Source: three-view drawing plus pictorial views. Frame: mm from the lowest corner of the part. Give positions to 0.01 mm unless a question says otherwise; leave off trailing zeros. Order: outer loops, then holes, each group sorted by start corner. A loop starts at its lowest first (then second) coordinate and runs counter-clockwise, first axis right, second up. Notation, with made-up numbers: M 72.25,37.5 L 125.25,37.5 A12 ccw 125.25,49.5 Z; hole C -30,80.25 d8. An arc over 180 degrees is marked long. Use CSV: the item, a comma, the result in double quotes. Start each with the question number.
Item 1: First-contact query: pin 1 (1.5 mm diameter, centred on y = 3, z = 27, fed in from +X); pin 2 (2 mm diameter, centred on x = 109.5, z = 37.5, fed in from -Y). Flat tips, straight axial feed; report the tip coordinate or a pass-through.
Item 2: Ray query, probe 1 along Y at (x, z) = (116, 39.5); probe 2 along X at (y, z) = (4, 17); probe 3 along Y at (x, z) = (21, 33). Return the intervals inside material, ascending. Write a range as from..to.
Item 3: Pull-direction query (Y, two-part tool) for the marked faces 1, 2 and 3; classes: +Y half, -Y half, draft (parallel to the pull), parting line (faces both ways), or undercut.
Item 4: Section query D-D on x = 126. Return loops of the section in (y, z).
Item 5: Section query C-C on z = 38.5. Return loops of the section in (x, y).
Item 6: Section query B-B on z = 12.5. Return loops of the section in (x, y).
Item 7: Section query A-A on x = 87.5. Return loops of the section in (y, z), and give its area (3 significant figures).
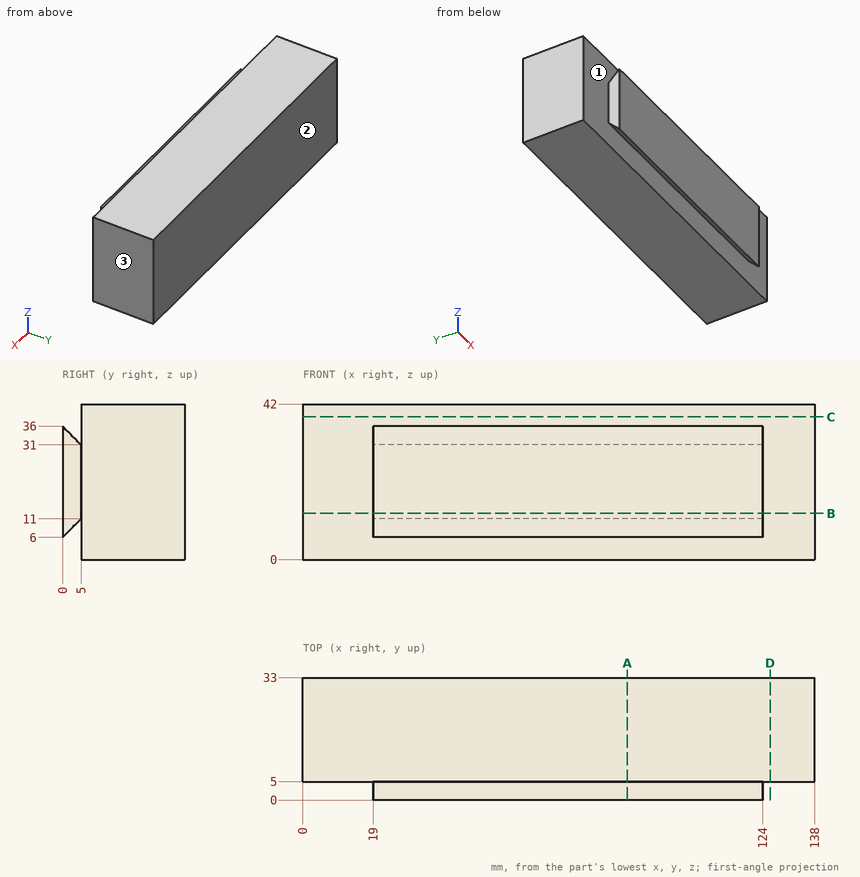
Verdict:
1,pin 1,"x = 124"
1,pin 2,"y = 5"
2,probe 1,"5..33"
2,probe 2,"19..124"
2,probe 3,"0..3, 5..33"
3,face 1,"undercut"
3,face 2,"+Y half"
3,face 3,"draft"
4,outline,"M 5,0 L 33,0 L 33,42 L 5,42 Z"
5,outline,"M 0,5 L 138,5 L 138,33 L 0,33 Z"
6,outline,"M 0,5 L 19,5 L 19,0 L 124,0 L 124,5 L 138,5 L 138,33 L 0,33 Z"
7,outline,"M 0,6 L 5,11 L 5,0 L 33,0 L 33,42 L 5,42 L 5,31 L 0,36 Z"
7,area,"1,300 mm2"
